Work out the finished part from the listing and answer in its coordinate system (mm). Face numbers are marked on the shaded views. A direction names the side the tool comes from. Coordinates: 2 decimals unless noted, no trailing zeros. Order: outer loops, then holes, each group sorted by start corner. A loop starts at its lowest first (then second) coordinate and runs counter-clockwise, first axis right, second up. Notation, with made-up numbers: M -21.5,40.25 L 1.5,40.25 A15 ccw 1.5,48.25 Z; hole C 37.5,78 d4. An arc over 180 degrees is marked long. Use a Markdown table: item, result.
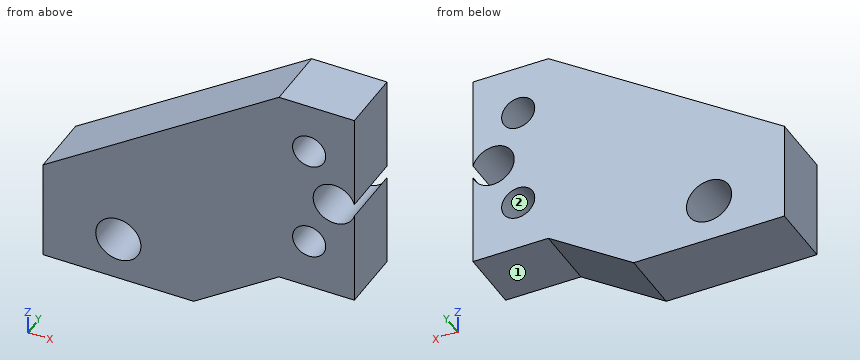
from build123d import *

# Parameters (mm, degrees)
BOSS_EXTRUDE1_DEPTH   = 3.175
M4_CLEARANCE_HOLE1_D  = 4.5
M4X0_7_TAPPED_HOLE1_D = 3.3
M5X0_8_TAPPED_HOLE1_D = 4.2


with BuildPart() as part:
    # Sketch1 → Boss-Extrude1 (new body, symmetric)
    with BuildSketch(Plane(origin=(0, 0, 0), x_dir=(1, 0, 0), z_dir=(0, 1, 0))):
        Polygon((0, 0), (0, 20), (-7.5, 20), (-16, 25.666666667), (-31, 25.666666667), (-31, 15.666666667), (-7.5, 0), align=None)
    extrude(amount=BOSS_EXTRUDE1_DEPTH, both=True)

    # M4 Clearance Hole1 (through all)
    with Locations(Plane(origin=(0, 3.175, 0), x_dir=(1, 0, 0), z_dir=(0, 1, 0))):
        with Locations((-23.5, 21.364471274)):
            Hole(M4_CLEARANCE_HOLE1_D / 2)

    # M4x0.7 Tapped Hole1 (through all)
    with Locations(Plane(origin=(0, 3.175, 0), x_dir=(1, 0, 0), z_dir=(0, 1, 0))):
        with Locations((-4.500000447, 15), (-4.500000447, 5)):
            Hole(M4X0_7_TAPPED_HOLE1_D / 2)

    # M5x0.8 Tapped Hole1 (through all)
    with Locations(Plane(origin=(0, 3.175, 0), x_dir=(1, 0, 0), z_dir=(0, 1, 0))):
        with Locations((-2, 10)):
            Hole(M5X0_8_TAPPED_HOLE1_D / 2)


solid = part.part
(1) Straight lines are drawn through the part: L1, parallel to Z at x = -4.5, y = -0.75; L2, parallel to Z at x = -2, y = -0.5; L3, parallel to X at y = -2.25, z = -22.5. For each, find the intervals that lie inside material, in ascending order.
Conclusion:
| item | result |
|---|---|
| L1 | -20 to -16.65, -13.35 to -6.65, -3.35 to 0 |
| L2 | -20 to -12.1, -7.9 to 0 |
| L3 | -31 to -25.44, -21.56 to -11.25 |
(2) Given P1, Ø2.5, axis at x = -4.5, z = -15, coming from the +Y side; P2, Ø5, axis at x = -2, z = -10, coming from the +Y side (3 decimals); P3, Ø1, axis at y = -2, z = -5.5, coming from the -X side, each flat-ended and moving along its own axis, determine where each tip first touches the part or whether it passes through.
Conclusion:
| item | result |
|---|---|
| P1 | through |
| P2 | y = 3.175 |
| P3 | x = -16.5 |
(3) A cutting plane is placed at D-D (z = -16). Determine the outline of the cut face in (x, y) (3 decimals), then the cut area to 3 significant figures.
Conclusion:
| item | result |
|---|---|
| outline | M -31,-3.175 L -5.812,-3.175 L -5.812,3.175 L -31,3.175 Z; M -3.188,-3.175 L 0,-3.175 L 0,3.175 L -3.188,3.175 Z |
| area | 180 mm2 |
(4) A cutting plane is placed at C-C (y = -0.5). Determine the outline of the cut face in (x, z).
Conclusion:
| item | result |
|---|---|
| outline | M -31,-25.67 L -16,-25.67 L -7.5,-20 L 0,-20 L 0,-10.64 A2.1 cw long 0,-9.36 L 0,0 L -7.5,0 L -31,-15.67 Z; hole C -23.5,-21.36 d4.5; hole C -4.5,-15 d3.3; hole C -4.5,-5 d3.3 |
(5) A cutting plane is placed at A-A (x = -4.5). Determine the outline of the cut face in (y, z) (3 decimals), then the cut area to 3 significant figures.
Conclusion:
| item | result |
|---|---|
| outline | M -3.175,-20 L 3.175,-20 L 3.175,-16.65 L -3.175,-16.65 Z; M -3.175,-13.35 L 3.175,-13.35 L 3.175,-6.65 L -3.175,-6.65 Z; M -3.175,-3.35 L 3.175,-3.35 L 3.175,0 L -3.175,0 Z |
| area | 85.1 mm2 |
(6) Which of the six approach directions +Z, -Z, +X, -X, +Y, -Y give full straight-line access (tool end or side, diameter ignored) to the marked faces 1 and 2?
Conclusion:
| item | result |
|---|---|
| face 1 | -Z, +X, +Y, -Y |
| face 2 | +Y, -Y |
(7) A cutting plane is placed at B-B (z = -5). Determine the outline of the cut face in (x, y) (3 decimals).
Conclusion:
| item | result |
|---|---|
| outline | M -15,-3.175 L -6.15,-3.175 L -6.15,3.175 L -15,3.175 Z; M -2.85,-3.175 L 0,-3.175 L 0,3.175 L -2.85,3.175 Z |
